Can you work these out from the model? Positions are in its coordinate system, mm. A direction names the side the tool comes from. Round coordinates to 2 decimals unless told otherwise and drop trailing zeros. Order: outer loops, then holes, each group sorted by start corner. A loop starts at its lowest first (then second) coordinate and runs counter-clockwise, first axis right, second up.
from build123d import *

# Parameters (mm, degrees)
SKETCH1_W           = 5
SKETCH1_H           = 3.8
BOSS_EXTRUDE1_DEPTH = 6
BOSS_EXTRUDE2_DEPTH = 5


with BuildPart() as part:
    # Sketch1 → Boss-Extrude1 (new body)
    with BuildSketch(Plane(origin=(0, 0, 0), x_dir=(1, 0, 0), z_dir=(0, 1, 0))):
        Polygon((12.5, 8.25), (12.5, 9.15), (-17.5, 9.15), (-17.5, -9.15), (12.5, -9.15), (12.5, -8.25), (12.5, -4.45), (12.5, -1.9), (12.5, 1.9), (12.5, 4.45), (17.5, 4.45), (17.5, 8.25), align=None)
        with Locations((15, 0)):
            Rectangle(SKETCH1_W, SKETCH1_H)
        with Locations((15, -6.35)):
            Rectangle(SKETCH1_W, SKETCH1_H)
    extrude(amount=BOSS_EXTRUDE1_DEPTH)

    # Sketch2 → Boss-Extrude2 (add)
    with BuildSketch(Plane(origin=(0, 0, 0), x_dir=(1, 0, 0), z_dir=(0, 1, 0))):
        Polygon((-17.5, 0), (-17.5, 9.15), (-27.5, 6), (-27.5, 0), align=None)
        Polygon((-17.5, -9.15), (-17.5, 0), (-27.5, 0), (-27.5, -6), align=None)
    extrude(amount=BOSS_EXTRUDE2_DEPTH)


solid = part.part
(1) I'm going to push flat-ended pins straight in: pin 1 Ø0.7 at (y, z) = (4, -9) entering from +X; pin 2 Ø2.5 at (x, y) = (16, 4.5) entering from +Z; pin 3 Ø1.1 at (y, z) = (5.5, -4) entering from -X; pin 4 Ø2.5 at (x, y) = (15.5, 4.5) entering from -Z. Where does each tip first touch, or does it pass through?
(2) I want a section at C-C, the plane z = 3.75. List the corners of the cut face in (x, y) for me, plus the area to 3 significant figures.
(3) I want a section at A-A, the plane y = 3.9. List the corners of the cut face in (x, z) for me.
(4) I want a section at D-D, the plane x = -22.5. List the corners of the cut face in (y, z) for me (3 decimals), plus the area to 4 significant figures.
(5) If we mould it in two halves opening along Z, with no side actions, what happens to faces 6 (the face through (12.5, 3, -9)), 7 (the face through (15, 3, 1.9)), 8 (the face through (12.5, 3, -3)), 9 (the face through (-3, 3, 9.15))? For each: pulls with the +Z half, pulls with the -Z half, needs draft (parallel to the pull), parting line crosses it, or undercut.
(6) Please list where these lines run through material, in increasing order: probe 1 along Z at (x, y) = (14, 4.45); probe 2 along X at (y, z) = (3.75, -4); probe 3 along X at (y, z) = (5.15, -2.25).
(7) On a 3-axis mill with a long thin cutter (end or side, diameter ignored), from which of +Z, -Z, +X, -X, +Y, -Y can I reach the whole of each face in a straight line? I mean faces 1 (the face through (15, 3, -4.45)), 2 (the face through (0, 6, 0)), 3 (the face through (-23, 5, 0)), 4 (the face through (-22.43, 2.465, -7.597)), 5 (the face through (15, 3, 8.25)). Say none if no direction works.
(8) I want a section at B-B, the plane z = 1.5. List the corners of the cut face in (x, y) for me.
Ans:
1. pin 1: stops at x = 12.5
1. pin 2: stops at z = 8.25
1. pin 3: stops at x = -27.5
1. pin 4: stops at z = -8.25
2. outline: (-27.5, 0) - (12.5, 0) - (12.5, 6) - (-17.5, 6) - (-17.5, 5) - (-27.5, 5) - close
2. area: 230 mm2
3. outline: (-27.5, -6) - (-17.5, -9.15) - (12.5, -9.15) - (12.5, -8.25) - (17.5, -8.25) - (17.5, -4.45) - (12.5, -4.45) - (12.5, -1.9) - (17.5, -1.9) - (17.5, 1.9) - (12.5, 1.9) - (12.5, 4.45) - (17.5, 4.45) - (17.5, 8.25) - (12.5, 8.25) - (12.5, 9.15) - (-17.5, 9.15) - (-27.5, 6) - close
4. outline: (0, -7.575) - (5, -7.575) - (5, 7.575) - (0, 7.575) - close
4. area: 75.75 mm2
5. face 6: needs draft
5. face 7: undercut
5. face 8: undercut
5. face 9: pulls with the +Z half
6. probe 1: z = -8.25 to -4.45, -1.9 to 1.9, 4.45 to 8.25
6. probe 2: x = -27.5 to 12.5
6. probe 3: x = -17.5 to 12.5
7. face 1: +X, +Y, -Y
7. face 2: +Z, -Z, +X, -X, +Y
7. face 3: +Z, -Z, -X, +Y
7. face 4: -Z, -X, +Y, -Y
7. face 5: +Z, +X, +Y, -Y
8. outline: (-27.5, 0) - (17.5, 0) - (17.5, 6) - (-17.5, 6) - (-17.5, 5) - (-27.5, 5) - close
